The listing builds one solid part. Answer for the finished solid, in the listing's coordinates (mm). Face numbers are marked on the shaded views. Give positions to 0.01 mm unless a question says otherwise; leave off trailing zeros. Order: outer loops, then holes, each group sorted by start corner. A loop starts at its lowest first (then second) coordinate and runs counter-clockwise, first axis right, second up. Notation, with made-up numbers: (-10, 88.5) -> (18, 88.5) arc R31 cw to (18, 116.5) -> close; hole circle Ø2 at (15.5, -9). An arc over 180 degrees is marked (long way). Write item = value, one per line. Start each with the question number.
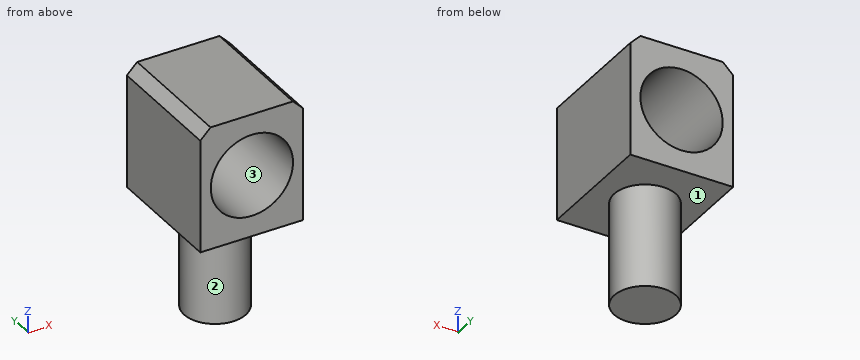
```python
from build123d import *

# Parameters (mm, degrees)
CROQUIS1_W              = 10
CROQUIS1_H              = 12
CROQUIS1_R              = 4
SALIENTE_EXTRUIR1_DEPTH = 12
CHAFL_N1_SIZE           = 1
CROQUIS2_R              = 3
SALIENTE_EXTRUIR2_DEPTH = 10


with BuildPart() as part:
    # Croquis1 → Saliente-Extruir1 (new body)
    with BuildSketch(Plane(origin=(0, 0, 0), x_dir=(1, 0, 0), z_dir=(0, 1, 0))):
        with Locations((5, -6)):
            Rectangle(CROQUIS1_W, CROQUIS1_H)
        with Locations((5.016573561, -6)):
            Circle(CROQUIS1_R, mode=Mode.SUBTRACT)
    extrude(amount=SALIENTE_EXTRUIR1_DEPTH)

    # Chaflán1
    chafl_n1_edges = [part.edges().sort_by_distance(p)[0] for p in [
        (10, 6, 12),
        (0, 6, 12),
    ]]
    chamfer(chafl_n1_edges, length=CHAFL_N1_SIZE)

    # Croquis2 → Saliente-Extruir2 (add)
    with BuildSketch(Plane(origin=(0, 0, 0), x_dir=(-1, 0, 0), z_dir=(0, 0, -1))):
        with Locations((-5, 6)):
            Circle(CROQUIS2_R)
    extrude(amount=SALIENTE_EXTRUIR2_DEPTH)


solid = part.part
```
Item 1: A cutting plane is placed at D-D, the plane y = 2.5. Write down the section's boundary in (x, z).
Item 2: Consider L1, parallel to Z at x = 5, y = 10.5; L2, parallel to X at y = 6.5, z = 6; L3, parallel to Z at x = 1.75, y = 3.5. Determine where each line is inside the solid, lowest interval first. Write a range as from..to.
Item 3: A cutting plane is placed at A-A, the plane z = 6. Write down the section's boundary in (x, y).
Item 4: A cutting plane is placed at B-B, the plane y = 6. Write down the section's boundary in (x, z), plus the area to 3 significant figures.
Item 5: A cutting plane is placed at C-C, the plane x = 5. Write down the section's boundary in (y, z), plus the area to 3 significant figures.
Item 6: The mould has two halves that part along X. Classify the marked faces 1, 2 and 3: +X half, -X half, draft (parallel to the pull), parting line (faces both ways), or undercut.
Check values:
q1.outline = (0, 0) -> (10, 0) -> (10, 11) -> (9, 12) -> (1, 12) -> (0, 11) -> close; hole circle Ø8 at (5.02, 6)
q2.L1 = 0..2, 10..12
q2.L2 = 0..1.02, 9.02..10
q2.L3 = 0..3.69, 8.31..12
q3.outline = (0, 0) -> (1.02, 0) -> (1.02, 12) -> (0, 12) -> close; (9.02, 0) -> (10, 0) -> (10, 12) -> (9.02, 12) -> close
q4.outline = (0, 0) -> (2, 0) -> (2, -10) -> (8, -10) -> (8, 0) -> (10, 0) -> (10, 11) -> (9, 12) -> (1, 12) -> (0, 11) -> close; hole circle Ø8 at (5.02, 6)
q4.area = 129 mm^2
q5.outline = (0, 0) -> (3, 0) -> (3, -10) -> (9, -10) -> (9, 0) -> (12, 0) -> (12, 2) -> (0, 2) -> close; (0, 10) -> (12, 10) -> (12, 12) -> (0, 12) -> close
q5.area = 108 mm^2
q6.face_1 = draft
q6.face_2 = parting line
q6.face_3 = undercut
